Could you check a few things on this model? Use its own coordinates, in mm. A direction names the side the tool comes from. Give positions to 0.01 mm unless a question says otherwise; leave off trailing zeros. Order: outer loops, then holes, each group sorted by start corner. A loop starts at its lowest first (then second) coordinate and runs counter-clockwise, first axis right, second up. Notation, with made-up numbers: (-37, 19.25) - (-14, 19.25) arc R27 cw to (-14, 56.25) - close; hole circle Ø1 at (-35.75, -33.75). An arc over 180 degrees is marked (long way). Put each result on its own line as item: value.
Autodesk Inventor part; units mm, degrees
ref_plane "YZ Plane" through (0, 0, 0) normal (1, 0, 0) x (0, 1, 0)
ref_plane "XZ Plane" through (0, 0, 0) normal (0, 1, 0) x (-1, 0, 0)
ref_plane "XY Plane" through (0, 0, 0) normal (0, 0, 1) x (1, 0, 0)
sketch "Sketch1" plane through (0, 0, 0) normal (0, 0, 1) x (1, 0, 0)
  line L0 (50.8, 0) -> (50.8, 1.2)
  line L1 (50.8, 1.2) -> (0, 1.2)
  line L2 (0, 1.2) -> (0, 0)
  line L3 (0, 0) -> (1.2, 0) construction
  line L4 (1.2, 0) -> (1.2, -7.6054) construction
  line L5 (1.2, -7.6054) -> (0, -7.6054) construction
  line L6 (0, -7.6054) -> (0, 0) construction
  line L7 (50.8, 0) -> (49.6, 0) construction
  line L8 (49.6, 0) -> (49.6, -9.5013) construction
  line L9 (49.6, -9.5013) -> (50.8, -9.5013) construction
  line L10 (50.8, -9.5013) -> (50.8, 0) construction
  line L11 (1.2, 0) -> (1.2, -2) construction
  line L12 (1.2, -1) -> (2.614, -1) construction
  line L13 (1.2, -2) -> (2.614, -1)
  line L14 (1.2, 0) -> (2.614, -1)
  line L15 (1.2, -2) -> (1.2, -2.6)
  line L16 (1.2, -2.6) -> (49.6, -2.6)
  line L17 (49.6, -2.6) -> (49.6, -2)
  line L18 (49.6, -2) -> (49.6, 0) construction
  line L19 (49.6, -1) -> (48.186, -1) construction
  line L20 (49.6, -2) -> (48.186, -1)
  line L21 (49.6, 0) -> (48.186, -1)
  line L22 (0, 0) -> (1.2, 0)
  line L23 (49.6, 0) -> (50.8, 0)
  dimension "Width" = 50.8
  dimension "Thickness" = 1.2
  dimension "Leftwall" = 1.2
  dimension "Rightwall" = 1.2
  dimension "LTheight" = 2
  dimension "LTwidth" = 1.414
  dimension "BThickness" = 0.6
  dimension "BThicknessR" = 0.6
  dimension "RTWidth" = 1.414
extrude "Extrusion1" add sketch "Sketch1" along normal blind 50
equation "\"Rightwall\" = Leftwall"
equation "\"BThicknessR\" = BThickness"
equation "\"RTWidth\" = LTwidth"
properties part number "channel_lid"
1) If I drill on line 1 (Y direction, x = 2, z = 8.5); line 2 (X direction, y = -2.25, z = 5); line 3 (X direction, y = -0.1, z = 29), over which ranges is the centre line in solid material (lowest first)? Write a range as [from, to].
Filled in:
line 1: y = [-2.6, -1.43], [-0.57, 1.2]
line 2: x = [1.2, 49.6]
line 3: x = [1.34, 49.46]
2) Which directions (+Z, -Z, +X, -X, +Y, -Y) give clear straight access to the entire face, cutting with the end or side of a thin tool? Please do faces 1 (the flat face through (25, -2.6, 25)), 2 (the flat face through (1, 0, 25)), 3 (the flat face through (48.903, -0.493, 24.65)).
Filled in:
face 1: +Z, -Z, +X, -X, -Y
face 2: +Z, -Z, -X, -Y
face 3: +Z, -Z, +X
3) Suppose I cut it at A-A, the plane z = 30.5. List the corners of the cut face in (x, y) for me.
Filled in:
outline: (0, 0) - (1.2, 0) - (2.61, -1) - (1.2, -2) - (1.2, -2.6) - (49.6, -2.6) - (49.6, -2) - (48.19, -1) - (49.6, 0) - (50.8, 0) - (50.8, 1.2) - (0, 1.2) - close
4) We'd pull the mould along Y, two halves only. Please class faces 4 (the flat face through (48.903, -1.507, 24.65)), 5 (the flat face through (26, 1.2, 25)), 6 (the flat face through (1.897, -0.493, 24.65)), 7 (the flat face through (50, 0, 25)): pulls with the +Y half, pulls with the -Y half, needs draft (parallel to the pull), parting line crosses it, or undercut.
Filled in:
face 4: undercut
face 5: pulls with the +Y half
face 6: undercut
face 7: pulls with the -Y half
5) I'm going to push a flat-ended pin straight in: pin 1 (1.3 mm diameter, centred on x = 50.5, z = 18, fed in from -Y). Where does the tip first touch, or does it pass through?
Filled in:
pin 1: stops at y = 0
